Verification items for the finished model (mm, model axes). A direction names the side the tool comes from. Give positions to 0.01 mm unless a question says otherwise; leave off trailing zeros. Loops run counter-clockwise (first coordinate to the right, second up) from the corner with the lowest first, then second, coordinate; pieces in that order, holes last. Notation, with made-up numbers: M 41.25,-39 L 98.25,-39 A34 cw 98.25,-2 Z; hole C 40.25,-17.5 d3. An arc over 180 degrees is marked long. Use CSV: the item, a comma, the result in double quotes.
from build123d import *

# Parameters (mm, degrees)
SKETCH4_R           = 10
BOSS_EXTRUDE1_DEPTH = 20
SKETCH5_R           = 10
BOSS_EXTRUDE2_DEPTH = 15
BOSS_EXTRUDE4_START = 10
SKETCH6_R           = 15
SKETCH6_R_2         = 10
BOSS_EXTRUDE4_DEPTH = 10
BOSS_EXTRUDE6_START = -15
SKETCH10_R          = 10
BOSS_EXTRUDE6_DEPTH = 15
SKETCH11_R          = 15
SKETCH11_R_2        = 10
BOSS_EXTRUDE7_DEPTH = 10
SKETCH12_R          = 25
BOSS_EXTRUDE8_DEPTH = 45
SKETCH14_R          = 20
CUT_EXTRUDE3_DEPTH  = 7
CUT_EXTRUDE3_DRAFT  = -45


with BuildPart() as part:
    # Sketch4 → Boss-Extrude1 (new body)
    with BuildSketch(Plane(origin=(0, 0, 0), x_dir=(1, 0, 0), z_dir=(0, 1, 0))):
        with BuildLine():
            Line((-77.28011811, -56.673598022), (-77.28011811, 23.326401978))
            Line((-77.28011811, 23.326401978), (-16.966387776, 23.326401978))
            ThreePointArc((-16.966387776, 23.326401978), (-3.737631221, 28.326401978), (2.876747057, 40.826401978))
            ThreePointArc((2.876747057, 40.826401978), (12.736944948, 55.656750215), (30.512681706, 56.745747))
            Line((30.512681706, 56.745747), (160.512681706, 1.745747))
            ThreePointArc((160.512681706, 1.745747), (172.71988189, -16.673598022), (160.512681706, -35.092943043))
            Line((160.512681706, -35.092943043), (30.512681706, -90.092943043))
            ThreePointArc((30.512681706, -90.092943043), (12.736944948, -89.003946259), (2.876747057, -74.173598022))
            ThreePointArc((2.876747057, -74.173598022), (-3.737631221, -61.673598022), (-16.966387776, -56.673598022))
            Line((-16.966387776, -56.673598022), (-77.28011811, -56.673598022))
        make_face()
        with Locations(Location((-57.28011811, -16.673598022, 0), (0, 0, 270))):
            Circle(SKETCH4_R, mode=Mode.SUBTRACT)
    extrude(amount=BOSS_EXTRUDE1_DEPTH)

    # Sketch5 → Boss-Extrude2 (add)
    with BuildSketch(Plane.XY.offset(56.673598022)):
        with BuildLine():
            Line((-77.28011811, 20), (-77.28011811, 60))
            ThreePointArc((-77.28011811, 60), (-60.595178298, 79.723345962), (-38.379080515, 66.538407896))
            Line((-38.379080515, 66.538407896), (-22.28011811, 20))
            Line((-22.28011811, 20), (-77.28011811, 20))
        make_face()
        with Locations((-57.28011811, 60)):
            Circle(SKETCH5_R, mode=Mode.SUBTRACT)
    extrude(amount=-BOSS_EXTRUDE2_DEPTH)

    # Sketch6 → Boss-Extrude4 (add)
    with BuildSketch(Plane.XY.offset(56.673598022).offset(BOSS_EXTRUDE4_START)):
        with Locations(Location((-57.28011811, 60, 0), (0, 0, 180))):
            Circle(SKETCH6_R)
        with Locations((-57.28011811, 60)):
            Circle(SKETCH6_R_2, mode=Mode.SUBTRACT)
    extrude(amount=-BOSS_EXTRUDE4_DEPTH)

    # Sketch10 → Boss-Extrude6 (add)
    with BuildSketch(Plane(origin=(0, 0, -23.326401978), x_dir=(-1, 0, 0), z_dir=(0, 0, -1)).offset(BOSS_EXTRUDE6_START)):
        with BuildLine():
            Line((22.28011811, 20), (38.379080515, 66.538407896))
            ThreePointArc((38.379080515, 66.538407896), (58.842761472, 79.938860191), (76.96898439, 63.514049605))
            Line((76.96898439, 63.514049605), (77.28011811, 20))
            Line((77.28011811, 20), (22.28011811, 20))
        make_face()
        with Locations(Location((57.28011811, 60, 0), (0, 0, 180))):
            Circle(SKETCH10_R, mode=Mode.SUBTRACT)
    extrude(amount=BOSS_EXTRUDE6_DEPTH)

    # Sketch11 → Boss-Extrude7 (add)
    with BuildSketch(Plane(origin=(0, 0, -23.326401978), x_dir=(-1, 0, 0), z_dir=(0, 0, -1))):
        with Locations((57.28011811, 60)):
            Circle(SKETCH11_R)
        with Locations(Location((57.28011811, 60, 0), (0, 0, 180))):
            Circle(SKETCH11_R_2, mode=Mode.SUBTRACT)
    extrude(amount=BOSS_EXTRUDE7_DEPTH)

    # Sketch12 → Boss-Extrude8 (add)
    with BuildSketch(Plane(origin=(0, 20, 0), x_dir=(1, 0, 0), z_dir=(0, 1, 0))):
        with Locations(Location((22.71988189, -16.673598022, 0), (0, 0, 90))):
            Circle(SKETCH12_R)
    extrude(amount=BOSS_EXTRUDE8_DEPTH)


with BuildPart() as cut_extrude3_tool:
    # Sketch14 → Cut-Extrude3 (with draft: the straight prism first)
    with BuildSketch(Plane(origin=(0, 65, 0), x_dir=(1, 0, 0), z_dir=(0, 1, 0))):
        with Locations((22.71988189, -16.673598022)):
            Circle(SKETCH14_R)
    extrude(amount=-CUT_EXTRUDE3_DEPTH)
    # Cut-Extrude3: the draft: its side faces are tilted about the plane it starts from
    cut_extrude3_sides = [cut_extrude3_tool.faces().sort_by_distance(p)[0] for p in [
        (2.71988189, 61.5, 16.673598022),
    ]]
    draft(cut_extrude3_sides, Plane(origin=(0, 65, 0), x_dir=(1, 0, 0), z_dir=(0, 1, 0)), CUT_EXTRUDE3_DRAFT)


with BuildPart() as part_1:
    add(part.part)

    # Cut-Extrude3: cut by cut_extrude3_tool
    add(cut_extrude3_tool.part, mode=Mode.SUBTRACT)


solid = part_1.part
(1) Section check C-C on y = 29.5. Record the cut outline in (x, z).
Calculated:
outline,"M -77.28,41.67 L -25.57,41.67 L -25.57,56.67 L -77.28,56.67 Z; M -77.21,-23.33 L -25.57,-23.33 L -25.57,-8.33 L -77.21,-8.33 Z; C 22.72,16.67 d50"
(2) Section check A-A on z = 59.5. Record the cut outline in (x, y), plus the area to 3 significant figures.
Calculated:
outline,"C -57.28,60 d30; M -6.72,0 L 102.82,0 L 102.82,20 L -6.72,20 Z; hole C -57.28,60 d20"
area,"2,580 mm²"
(3) Mould release check, pull along X, two halves, no side actions. Record for faces 1 (the flat face through (-30.2, 42.9, -15.7)), 2 (the cylindrical face through (-47.365, 9.86, 15.372)), 3 (the flat face through (-56, 44, 41.674)), 4 (the cylindrical face through (-65.22, 66.08, -20.65)): released by +X, released by -X, zero draft, split by the parting line, or undercut.
Calculated:
face 1,"released by +X"
face 2,"undercut"
face 3,"zero draft"
face 4,"undercut"
(4) Section check D-D on x = -13.5. Record the cut outline in (y, z).
Calculated:
outline,"M 0,-23.63 L 20,-23.63 L 20,56.98 L 0,56.98 Z"
(5) Depth check by flat-ended pin: pin 1 Ø16.5 at (x, y) = (-43.5, 63.5) entering from -Z; pin 2 Ø4 at (y, z) = (17, 37) entering from +X; pin 3 Ø6 at (y, z) = (34, -0.5) entering from -X; pin 4 Ø10 at (x, z) = (92.5, -40.5) entering from +Y. Enter the tip coordinate at first touch or a pass-through.
Calculated:
pin 1,"stops at z = -33.33"
pin 2,"stops at x = 160.73"
pin 3,"stops at x = 2.13"
pin 4,"passes through"
(6) Section check B-B on x = -52. Record the cut outline in (y, z), plus the area to 3 significant figures.
Calculated:
outline,"M 0,-23.33 L 45.96,-23.33 L 45.96,-33.33 L 51.51,-33.33 L 51.51,-8.33 L 20,-8.33 L 20,8.18 L 0,8.18 Z; M 0,25.17 L 20,25.17 L 20,41.67 L 51.51,41.67 L 51.51,66.67 L 45.96,66.67 L 45.96,56.67 L 0,56.67 Z; M 68.49,-33.33 L 74.04,-33.33 L 74.04,-23.33 L 79.29,-23.33 L 79.29,-8.33 L 68.49,-8.33 Z; M 68.49,41.67 L 79.29,41.67 L 79.29,56.67 L 74.04,56.67 L 74.04,66.67 L 68.49,66.67 Z"
area,"2,750 mm²"
(7) Tool access check on faces 5 (the flat face through (6, 65, 28)), 6 (the flat face through (49, 20, 16)), 7 (the flat face through (-56, 44, -8.326)), 8 (the flat face through (94.6, 9.86, -29.63)), 9 (the cylindrical face through (-64.2, 46.69, -28.26)). Record the directions out of +Z, -Z, +X, -X, +Y, -Y that give a thin tool (end or side, any length) a straight path to the whole face; none if there is none.
Calculated:
face 5,"+Z, -Z, +X, -X, +Y"
face 6,"+Y"
face 7,"-X, +Y"
face 8,"-Z, +X, +Y, -Y"
face 9,"-Z"
(8) Scan lines: L1, parallel to Y at x = -2.5, z = 27.5; L2, parallel to X at y = 57, z = -29; L3, parallel to Y at x = -51.5, z = -14. Record each from-to range of solid material in increasing order. Write a range as from..to.
Calculated:
L1,"y = 0..20"
L2,"x = -71.98..-66.82, -47.74..-42.58"
L3,"y = 0..51.84, 68.16..79.15"
